Source: CAD feature listing. Evaluate the final solid. Frame: model axes, mm. A direction names the side the tool comes from. Give positions to 0.01 mm unless a question says otherwise; leave off trailing zeros. Loops run counter-clockwise (first coordinate to the right, second up) from the corner with the lowest first, then second, coordinate; pieces in that order, holes last. Notation, with made-up numbers: M -2.5,82.5 L 44.5,82.5 A19 ccw 44.5,111.5 Z; hole C -25,-12 d4. An arc over 180 degrees is marked long. Put each result on its own line as item: value.
Autodesk Inventor part; units mm, degrees
ref_plane "YZ Plane" through (0, 0, 0) normal (1, 0, 0) x (0, 1, 0)
ref_plane "XZ Plane" through (0, 0, 0) normal (0, 1, 0) x (-1, 0, 0)
ref_plane "XY Plane" through (0, 0, 0) normal (0, 0, 1) x (1, 0, 0)
sketch "Sketch1" plane through (0, 0, 0) normal (0, 0, 1) x (1, 0, 0)
  circle A0 centre (-40, 0) radius 2.5
  arc A1 (-31.25, -10) -> (-30, -8.75) centre (-31.25, -8.75) ccw
  line L0 (-30, -3.6) -> (-30, -8.75)
  line L1 (-30.5, -3.1) -> (-30, -3.6)
  line L2 (-31.6, -3.1) -> (-30.5, -3.1)
  line L3 (-31.6, -5.5) -> (-31.6, -3.1)
  line L4 (-33.534, -5.5) -> (-31.6, -5.5)
  line L5 (-35.9, -3.134) -> (-33.534, -5.5)
  line L6 (-35.9, 3.134) -> (-35.9, -3.134)
  line L7 (-33.534, 5.5) -> (-35.9, 3.134)
  line L8 (-31.6, 5.5) -> (-33.534, 5.5)
  line L9 (-31.6, 3.1) -> (-31.6, 5.5)
  line L10 (-30.5, 3.1) -> (-31.6, 3.1)
  line L11 (-30, 3.6) -> (-30.5, 3.1)
  line L12 (-30, 8.75) -> (-30, 3.6)
  arc A2 (-30, 8.75) -> (-31.25, 10) centre (-31.25, 8.75) ccw
  line L13 (-36.4, 10) -> (-31.25, 10)
  line L14 (-36.9, 9.5) -> (-36.4, 10)
  line L15 (-36.9, 8.4) -> (-36.9, 9.5)
  line L16 (-34.5, 8.4) -> (-36.9, 8.4)
  line L17 (-34.5, 6.466) -> (-34.5, 8.4)
  line L18 (-36.866, 4.1) -> (-34.5, 6.466)
  line L19 (-43.134, 4.1) -> (-36.866, 4.1)
  line L20 (-45.5, 6.466) -> (-43.134, 4.1)
  line L21 (-45.5, 8.4) -> (-45.5, 6.466)
  line L22 (-43.1, 8.4) -> (-45.5, 8.4)
  line L23 (-43.1, 9.5) -> (-43.1, 8.4)
  line L24 (-43.6, 10) -> (-43.1, 9.5)
  line L25 (-48.75, 10) -> (-43.6, 10)
  arc A3 (-48.75, 10) -> (-50, 8.75) centre (-48.75, 8.75) ccw
  line L26 (-50, 3.6) -> (-50, 8.75)
  line L27 (-49.5, 3.1) -> (-50, 3.6)
  line L28 (-48.4, 3.1) -> (-49.5, 3.1)
  line L29 (-48.4, 5.5) -> (-48.4, 3.1)
  line L30 (-46.466, 5.5) -> (-48.4, 5.5)
  line L31 (-44.1, 3.134) -> (-46.466, 5.5)
  line L32 (-44.1, -3.134) -> (-44.1, 3.134)
  line L33 (-46.466, -5.5) -> (-44.1, -3.134)
  line L34 (-48.4, -5.5) -> (-46.466, -5.5)
  line L35 (-48.4, -3.1) -> (-48.4, -5.5)
  line L36 (-49.5, -3.1) -> (-48.4, -3.1)
  line L37 (-50, -3.6) -> (-49.5, -3.1)
  line L38 (-50, -8.75) -> (-50, -3.6)
  arc A4 (-50, -8.75) -> (-48.75, -10) centre (-48.75, -8.75) ccw
  line L39 (-43.6, -10) -> (-48.75, -10)
  line L40 (-43.1, -9.5) -> (-43.6, -10)
  line L41 (-43.1, -8.4) -> (-43.1, -9.5)
  line L42 (-45.5, -8.4) -> (-43.1, -8.4)
  line L43 (-45.5, -6.466) -> (-45.5, -8.4)
  line L44 (-43.134, -4.1) -> (-45.5, -6.466)
  line L45 (-36.866, -4.1) -> (-43.134, -4.1)
  line L46 (-34.5, -6.466) -> (-36.866, -4.1)
  line L47 (-34.5, -8.4) -> (-34.5, -6.466)
  line L48 (-36.9, -8.4) -> (-34.5, -8.4)
  line L49 (-36.9, -9.5) -> (-36.9, -8.4)
  line L50 (-36.4, -10) -> (-36.9, -9.5)
  line L51 (-31.25, -10) -> (-36.4, -10)
  circle A5 centre (0, 0) radius 2.5
  arc A6 (8.75, -10) -> (10, -8.75) centre (8.75, -8.75) ccw
  line L52 (10, -3.6) -> (10, -8.75)
  line L53 (9.5, -3.1) -> (10, -3.6)
  line L54 (8.4, -3.1) -> (9.5, -3.1)
  line L55 (8.4, -5.5) -> (8.4, -3.1)
  line L56 (6.466, -5.5) -> (8.4, -5.5)
  line L57 (4.1, -3.134) -> (6.466, -5.5)
  line L58 (4.1, 3.134) -> (4.1, -3.134)
  line L59 (6.466, 5.5) -> (4.1, 3.134)
  line L60 (8.4, 5.5) -> (6.466, 5.5)
  line L61 (8.4, 3.1) -> (8.4, 5.5)
  line L62 (9.5, 3.1) -> (8.4, 3.1)
  line L63 (10, 3.6) -> (9.5, 3.1)
  line L64 (10, 8.75) -> (10, 3.6)
  arc A7 (10, 8.75) -> (8.75, 10) centre (8.75, 8.75) ccw
  line L65 (3.6, 10) -> (8.75, 10)
  line L66 (3.1, 9.5) -> (3.6, 10)
  line L67 (3.1, 8.4) -> (3.1, 9.5)
  line L68 (5.5, 8.4) -> (3.1, 8.4)
  line L69 (5.5, 6.466) -> (5.5, 8.4)
  line L70 (3.134, 4.1) -> (5.5, 6.466)
  line L71 (-3.134, 4.1) -> (3.134, 4.1)
  line L72 (-5.5, 6.466) -> (-3.134, 4.1)
  line L73 (-5.5, 8.4) -> (-5.5, 6.466)
  line L74 (-3.1, 8.4) -> (-5.5, 8.4)
  line L75 (-3.1, 9.5) -> (-3.1, 8.4)
  line L76 (-3.6, 10) -> (-3.1, 9.5)
  line L77 (-8.75, 10) -> (-3.6, 10)
  arc A8 (-8.75, 10) -> (-10, 8.75) centre (-8.75, 8.75) ccw
  line L78 (-10, 3.6) -> (-10, 8.75)
  line L79 (-9.5, 3.1) -> (-10, 3.6)
  line L80 (-8.4, 3.1) -> (-9.5, 3.1)
  line L81 (-8.4, 5.5) -> (-8.4, 3.1)
  line L82 (-6.466, 5.5) -> (-8.4, 5.5)
  line L83 (-4.1, 3.134) -> (-6.466, 5.5)
  line L84 (-4.1, -3.134) -> (-4.1, 3.134)
  line L85 (-6.466, -5.5) -> (-4.1, -3.134)
  line L86 (-8.4, -5.5) -> (-6.466, -5.5)
  line L87 (-8.4, -3.1) -> (-8.4, -5.5)
  line L88 (-9.5, -3.1) -> (-8.4, -3.1)
  line L89 (-10, -3.6) -> (-9.5, -3.1)
  line L90 (-10, -8.75) -> (-10, -3.6)
  arc A9 (-10, -8.75) -> (-8.75, -10) centre (-8.75, -8.75) ccw
  line L91 (-3.6, -10) -> (-8.75, -10)
  line L92 (-3.1, -9.5) -> (-3.6, -10)
  line L93 (-3.1, -8.4) -> (-3.1, -9.5)
  line L94 (-5.5, -8.4) -> (-3.1, -8.4)
  line L95 (-5.5, -6.466) -> (-5.5, -8.4)
  line L96 (-3.134, -4.1) -> (-5.5, -6.466)
  line L97 (3.134, -4.1) -> (-3.134, -4.1)
  line L98 (5.5, -6.466) -> (3.134, -4.1)
  line L99 (5.5, -8.4) -> (5.5, -6.466)
  line L100 (3.1, -8.4) -> (5.5, -8.4)
  line L101 (3.1, -9.5) -> (3.1, -8.4)
  line L102 (3.6, -10) -> (3.1, -9.5)
  line L103 (8.75, -10) -> (3.6, -10)
  line L104 (-50, -10) -> (-50, 10)
  line L105 (10, 10) -> (10, -10)
  line L106 (-30, -10) -> (-30, 10)
  line L107 (-10, 10) -> (-10, -10)
  line L108 (-52.54, -12.54) -> (12.54, -12.54)
  line L109 (12.54, -12.54) -> (12.54, 12.54)
  line L110 (12.54, 12.54) -> (-52.54, 12.54)
  line L111 (-52.54, 12.54) -> (-52.54, -12.54)
  line L112 (10, -10) -> (-10, -10)
  line L113 (-30, -10) -> (-50, -10)
  line L114 (-50, 10) -> (-30, 10)
  line L115 (-10, 10) -> (10, 10)
  point P0 (0, 0)
extrude "Extrusion1" add sketch "Sketch1" against normal blind 7.62 contours L111 L110 L109 L108
sketch "Sketch2" plane through (0, 0, 0) normal (0, 0, 1) x (1, 0, 0)
  line L0 (-52.54, -12.54) -> (-52.54, 12.54)
  line L1 (12.54, -12.54) -> (12.54, 12.54)
  line L2 (-52.54, -12.54) -> (12.54, -12.54)
  line L3 (12.54, -12.54) -> (12.54, 12.54)
  line L4 (12.54, 12.54) -> (-52.54, 12.54)
  line L5 (-52.54, 12.54) -> (-52.54, -12.54)
  point P0 (0, 0)
extrude "Extrusion2" add sketch "Sketch2" along normal blind 6.35
sketch "Sketch3" plane through (12.54, -12.54, -7.62) normal (1, 0, 0) x (0, 0, -1)
  line L0 (0, 0) -> (-13.97, 0)
  line L1 (0, 25.08) -> (0, 0)
  line L2 (0, 25.08) -> (-13.97, 25.08)
  line L3 (-13.97, 0) -> (-13.97, 25.08)
  point P0 (-7.62, 12.54)
extrude "Extrusion3" add sketch "Sketch3" along normal blind 3.81
sketch "Sketch4" plane through (-52.54, -12.54, -7.62) normal (-1, 0, 0) x (0, 0, 1)
  line L0 (0, 25.08) -> (13.97, 25.08)
  line L1 (0, 0) -> (0, 25.08)
  line L2 (13.97, 0) -> (0, 0)
  line L3 (13.97, 25.08) -> (13.97, 0)
  point P0 (7.62, 12.54)
extrude "Extrusion4" add sketch "Sketch4" along normal blind 3.81
sketch "Sketch5" plane through (0, 0, -7.62) normal (0, 0, -1) x (-1, 0, 0)
  line L0 (-16.35, -12.54) -> (-16.35, 12.54)
  line L1 (56.35, -12.54) -> (-16.35, -12.54)
  line L2 (-16.35, 12.54) -> (-10, 12.54)
  line L3 (-10, 12.54) -> (-10, -12.54)
  line L4 (-10, -12.54) -> (-16.35, -12.54)
  line L5 (-16.35, -12.54) -> (-16.35, 12.54)
  line L6 (56.35, 12.54) -> (50, 12.54)
  line L7 (50, 12.54) -> (50, -12.54)
  line L8 (50, -12.54) -> (56.35, -12.54)
  line L9 (56.35, -12.54) -> (56.35, 12.54)
  line L10 (50, 10) -> (50, -10)
  line L11 (-10, -10) -> (-10, 10)
  line L12 (50, 12.54) -> (56.35, -12.54) construction
  line L13 (-16.35, 12.54) -> (56.35, 12.54) construction
  line L14 (-16.35, 12.54) -> (-10, -12.54) construction
  line L15 (-16.35, -10) -> (-10, -10)
  line L16 (-10, -10) -> (-10, 10)
  line L17 (-10, 10) -> (-16.35, 10)
  line L18 (-16.35, 10) -> (-16.35, -10)
  line L19 (-16.35, -10) -> (-10, 10) construction
  line L20 (-10, -10) -> (-16.35, 10) construction
  line L21 (50, -10) -> (56.35, -10)
  line L22 (56.35, -10) -> (56.35, 10)
  line L23 (56.35, 10) -> (50, 10)
  line L24 (50, 10) -> (50, -10)
  line L25 (50, -10) -> (56.35, 10) construction
  line L26 (56.35, -10) -> (50, 10) construction
  point P0 (0, 0)
  point P1 (-13.175, 0)
  point P2 (53.175, 0)
  dimension "d10" = 0
  dimension "d11" = 0
  dimension "d20" = 0
  dimension "d21" = 20
  dimension "d22" = 0
extrude "Extrusion5" add sketch "Sketch5" along normal blind 6.35 contours L0 L17 L3 L15 | L7 L23 L9 L21
sketch "Sketch6" plane through (-56.35, -12.54, -7.62) normal (-1, 0, 0) x (0, 0, 1)
  line L0 (0, 25.08) -> (13.97, 25.08)
  circle A0 centre (0, 12.54) radius 2.5
  line L1 (13.97, 25.08) -> (0, 25.08)
  line L2 (0, 25.08) -> (0, -0.9572)
  line L3 (-6.35, 2.54) -> (-6.35, 22.54)
  point P0 (7.62, 12.54)
  dimension "d14" = 5
  dimension "d23" = 6.35
extrude "Extrusion6" cut sketch "Sketch6" against normal through all
sketch "Sketch8" plane through (-10, -10, 0) normal (1, 0, 0) x (0, 0, -1)
  arc A0 (7.62, 12.5) -> (7.62, 7.5) centre (7.62, 10) ccw
  line L0 (7.62, 7.5) -> (7.62, 0)
  line L1 (7.62, 12.5) -> (7.62, 7.5)
  point P0 (0, 10)
extrude "Extrusion7" add sketch "Sketch8" against normal up to surface (20 mm away)
sketch "Sketch9" plane through (0, 0, 6.35) normal (0, 0, 1) x (1, 0, 0)
  line L0 (16.35, 12.54) -> (-56.35, 12.54) construction
  line L1 (-56.35, -12.54) -> (16.35, -12.54) construction
  line L2 (16.35, 12.54) -> (-56.35, -12.54) construction
  circle A0 centre (-20, 0) radius 2.75
  point P0 (0, 0)
  dimension "d24" = 5.5
extrude "Extrusion8" cut sketch "Sketch9" against normal blind 25.4
properties part number "cap"
1. Contact query for flat-ended pins moving along their axis: P1, Ø7.5, axis at x = -24, y = 2, coming from the -Z side; P2, Ø1.9, axis at x = -52.5, z = -11, coming from the +Y side; P3, Ø1.5, axis at x = 6, y = 6.5, coming from the -Z side; P4, Ø4.5, axis at x = -20, y = 0, coming from the +Z side. Output: stop coordinate, or through.
Found:
P1: z = -7.62
P2: y = 10
P3: z = 0
P4: through
2. Section query D-D (z = -6.5). Output: boundary loops of the cut face in (x, y), plus the area to 3 significant figures.
Found:
outline: M -56.35,-12.54 L 16.35,-12.54 L 16.35,-2.24 L 10,-2.24 L 10,-10 L -10,-10 L -10,10 L 10,10 L 10,2.24 L 16.35,2.24 L 16.35,12.54 L -56.35,12.54 L -56.35,2.24 L -50,2.24 L -50,10 L -30,10 L -30,-10 L -50,-10 L -50,-2.24 L -56.35,-2.24 Z; hole C -20,0 d5.5
area: 943 mm^2
3. Access query for faces 4 (the flat face through (13, 10, -11)), 5 (the flat face through (-30, 0, -4)), 6 (the flat face through (-19, -12.54, -1)). Directions: +Z, -Z, +X, -X, +Y, -Y. A direction counts if a zero-diameter tool reaches every point of the face in a straight line with its end or side. Return the directions, or none.
Found:
face 4: -Z, +X, -X, +Y
face 5: -Z
face 6: +Z, -Z, +X, -X, -Y
4. Draft query along Y for faces 1 (the flat face through (13, -10, -11)), 2 (the flat face through (-50, 2, -5)), 3 (the flat face through (-53, 10, -11)). Return one class per face: pulls with the +Y half, pulls with the -Y half, needs draft (parallel to the pull), parting line crosses it, or undercut.
Found:
face 1: pulls with the -Y half
face 2: undercut
face 3: pulls with the +Y half
5. Section query B-B (y = 0). Output: boundary loops of the cut face in (x, z), plus the area to 3 significant figures.
Found:
outline: M -56.35,-13.97 L -50,-13.97 L -50,-10.12 L -56.35,-10.12 Z; M -56.35,-5.12 L -50,-5.12 L -50,0 L -30,0 L -30,-7.62 L -22.75,-7.62 L -22.75,6.35 L -56.35,6.35 Z; M -17.25,-7.62 L -10,-7.62 L -10,0 L 10,0 L 10,-5.12 L 16.35,-5.12 L 16.35,6.35 L -17.25,6.35 Z; M 10,-13.97 L 16.35,-13.97 L 16.35,-10.12 L 10,-10.12 Z
area: 651 mm^2
6. Section query C-C (x = -45). Output: boundary loops of the cut face in (y, z), plus the area to 3 significant figures.
Found:
outline: M -12.54,-7.62 L -10,-7.62 L -10,0 L 10,0 L 10,-7.62 L 12.54,-7.62 L 12.54,6.35 L -12.54,6.35 Z
area: 198 mm^2
7. Material intervals for line 1 (X direction, y = -8, z = -3.75); line 2 (X direction, y = -6.25, z = -10.75); line 3 (Y direction, x = -42.5, z = -2.75), sorted ascending. Write a range as from..to.
Found:
line 1: -56.35..-50, -30..-10, 10..16.35
line 2: -56.35..-50, 10..16.35
line 3: -12.54..-10, 10..12.54
8. Section query A-A (x = -20). Output: boundary loops of the cut face in (y, z).
Found:
outline: M -12.54,-7.62 L -2.75,-7.62 L -2.75,6.35 L -12.54,6.35 Z; M 2.75,-7.62 L 12.54,-7.62 L 12.54,6.35 L 2.75,6.35 Z
